The drawing under review shows one solid part. Ordinate dimensions are in mm from its lowest x, y, z. Coordinates: 2 decimals unless noted, no trailing zeros. Loops run counter-clockwise (first coordinate to the right, second up) from the corner with the lowest first, then second, coordinate; pieces in that order, holes last. Notation, with made-up numbers: (50, -1) - (78, -1) arc R11 ccw to (78, 17) - close; hole circle Ø9 at (82, 54.25). An arc over 180 degrees is marked (long way). Answer as a JSON object with one key per item and string values. Group by question number.
Item 1: Mouldability with a two-part tool opening along Y and no side actions: class the marked faces 1, 2 and 3 as released by +Y, released by -Y, zero draft, split by the parting line, or undercut.
Item 2: We need section B-B (x = 25). Give the boundary of the cut face in (y, z).
Item 3: To check wall thickness, follow line 1 (Y direction, x = 26, z = 7); line 2 (Z direction, x = 25.5, y = 15); line 3 (Y direction, x = 30.5, z = 4). State the ranges of each line that lie inside material, in increasing order.
Item 4: Clearance check with flat-ended pins moving along their axes: pin 1 (3 mm diameter, centred on y = 37, z = 17.5, fed in from +X); pin 2 (4 mm diameter, centred on x = 15, y = 46, fed in from +Z); pin 3 (10 mm diameter, centred on x = 21.5, y = 20.5, fed in from +Z); pin 4 (25 mm diameter, centred on x = 21, z = 23.5, fed in from -Y). State where each tip first meets the part, or that it passes through.
Item 5: We need section A-A (z = 38.5). Give the boundary of the cut face in (x, y), then the cut area to 3 significant figures.
Item 6: We need section D-D (y = 57). Give the boundary of the cut face in (x, z), then the cut area to 3 significant figures.
Item 7: We need section C-C (x = 42.5). Give the boundary of the cut face in (y, z).
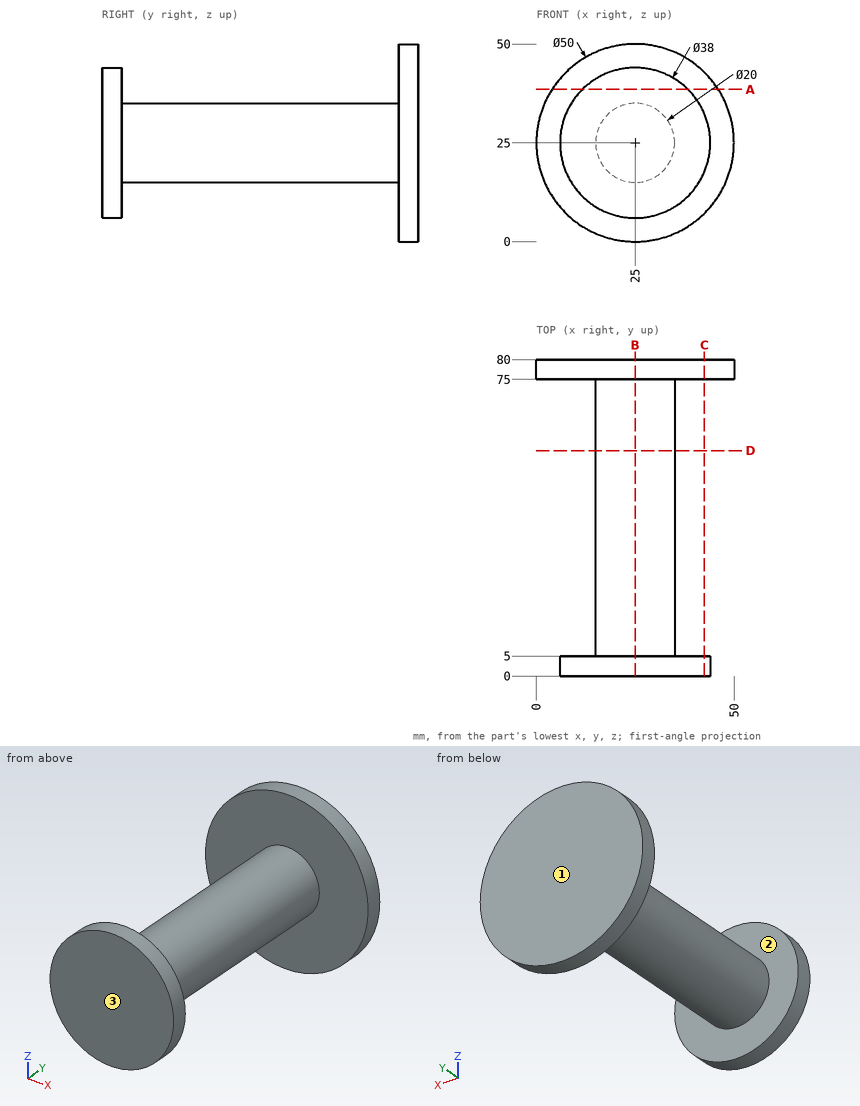
Check sheet entries:
{
 "1": {"face 1": "released by +Y", "face 2": "undercut", "face 3": "released by -Y"},
 "2": {"outline": "(0, 6) - (5, 6) - (5, 15) - (75, 15) - (75, 0) - (80, 0) - (80, 50) - (75, 50) - (75, 35) - (5, 35) - (5, 44) - (0, 44) - close"},
 "3": {"line 1": "y = 0 to 5, 75 to 80", "line 2": "z = 15.01 to 34.99", "line 3": "y = 75 to 80"},
 "4": {"pin 1": "stops at x = 33", "pin 2": "stops at z = 31", "pin 3": "stops at z = 35", "pin 4": "stops at y = 0"},
 "5": {"outline": "(3.96, 75) - (46.04, 75) - (46.04, 80) - (3.96, 80) - close; (11.63, 0) - (38.37, 0) - (38.37, 5) - (11.63, 5) - close", "area": "344 mm2"},
 "6": {"outline": "circle Ø20 at (25, 25)", "area": "314 mm2"},
 "7": {"outline": "(0, 17.6) - (5, 17.6) - (5, 32.4) - (0, 32.4) - close; (75, 7.15) - (80, 7.15) - (80, 42.85) - (75, 42.85) - close"}
}
